Autodesk Inventor part; units mm, degrees
ref_plane "YZ Plane" through (0, 0, 0) normal (1, 0, 0) x (0, 1, 0)
ref_plane "XZ Plane" through (0, 0, 0) normal (0, 1, 0) x (-1, 0, 0)
ref_plane "XY Plane" through (0, 0, 0) normal (0, 0, 1) x (1, 0, 0)
sketch "スケッチ1" plane through (0, 0, 0) normal (0, 0, 1) x (1, 0, 0)
  line L0 (0, 0) -> (90, 0)
  line L1 (90, 0) -> (90, 10)
  line L2 (90, 10) -> (0, 10)
  line L3 (0, 10) -> (0, 0)
  dimension "d0" = 90
  dimension "d1" = 10
extrude "押し出し1" add sketch "スケッチ1" along normal blind 2
sketch "スケッチ2" plane through (0, 0, 2) normal (0, 0, 1) x (1, 0, 0)
  line L0 (0, 10) -> (0, 0)
  line L1 (90, 0) -> (90, 10)
  line L2 (0, 0) -> (90, 0)
  point P0 (5, 5)
  point P1 (45, 5)
  point P2 (85, 5)
  dimension "d13" = 5
  dimension "d14" = 5
  dimension "d15" = 40
  dimension "d16" = 5
  dimension "d17" = 5
hole "穴1" at (5, 5, 2) at (45, 5, 2) at (85, 5, 2) direction (0, 0, -1) diameter 3 end through all
properties part number "長いほう"
Work out the finished part from the listing and answer in its coordinate system (mm). Round coordinates to 2 decimals unless told otherwise and drop trailing zeros. Write each loop counter-clockwise with the first axis right and the second up, starting at its lowest first coordinate (ties: lowest second). Pieces come first, ordered by that corner, then holes.
1) Flat-ended cylindrical pins translate along their axes: P1, Ø3, axis at x = 46.5, y = 3, coming from the -Z side; P2, Ø2.5, axis at x = 5, y = 5, coming from the +Z side. Find the tip coordinate at first contact, or state that the pin passes through.
2) A cutting plane is placed at A-A on y = 5. Determine the outline of the cut face in (x, z), and give its area (3 significant figures).
3) A cutting plane is placed at B-B on x = 5. Determine the outline of the cut face in (y, z).
4) Consider probe 1 along X at (y, z) = (5, 1.2); probe 2 along Y at (x, z) = (85, 0.9); probe 3 along X at (y, z) = (3.75, 1.55). Determine where each line is inside the solid, lowest interval first.
5) A cutting plane is placed at C-C on z = 0.85. Determine the outline of the cut face in (x, y).
6) Determine the mould class of faces 1 (the face through (44, 3, 0)), 2 (the face through (46, 10, 1)), 3 (the face through (3.99, 6.11, 0.99)), 4 (the face through (46.464, 5.325, 0.986)) for opening direction Y: pulls with the +Y half, pulls with the -Y half, needs draft (parallel to the pull), parting line crosses it, or undercut.
Entries:
1. P1: stops at z = 0
1. P2: passes through
2. outline: (0, 0) - (3.5, 0) - (3.5, 2) - (0, 2) - close; (6.5, 0) - (43.5, 0) - (43.5, 2) - (6.5, 2) - close; (46.5, 0) - (83.5, 0) - (83.5, 2) - (46.5, 2) - close; (86.5, 0) - (90, 0) - (90, 2) - (86.5, 2) - close
2. area: 162 mm2
3. outline: (0, 0) - (3.5, 0) - (3.5, 2) - (0, 2) - close; (6.5, 0) - (10, 0) - (10, 2) - (6.5, 2) - close
4. probe 1: x = 0 to 3.5, 6.5 to 43.5, 46.5 to 83.5, 86.5 to 90
4. probe 2: y = 0 to 3.5, 6.5 to 10
4. probe 3: x = 0 to 4.17, 5.83 to 44.17, 45.83 to 84.17, 85.83 to 90
5. outline: (0, 0) - (90, 0) - (90, 10) - (0, 10) - close; hole circle Ø3 at (5, 5); hole circle Ø3 at (45, 5); hole circle Ø3 at (85, 5)
6. face 1: needs draft
6. face 2: pulls with the +Y half
6. face 3: undercut
6. face 4: undercut
